from build123d import *

# Parameters (mm, degrees)
BASE_FLANGE1_DEPTH = 374.65
SKETCH6_R          = 3.3782
CUT_EXTRUDE1_DEPTH = 378.077201147
SKETCH7_R          = 4.3688
CUT_EXTRUDE2_DEPTH = 378.077201147
FILLET1_R          = 6.35


# Sheet-metal steps are written as plain solids
with BuildPart() as part:
    # Sketch1 → Base-Flange1 (new body)
    with BuildSketch(Plane(origin=(0, 0, 0), x_dir=(0, 0, -1), z_dir=(1, 0, 0))):
        with BuildLine():
            Line((0, 0), (25.4, 0))
            ThreePointArc((25.4, 0), (29.890128061, 1.859871939), (31.75, 6.35))
            Line((31.75, 6.35), (31.75, 31.75))
            Line((31.75, 31.75), (28.575, 31.75))
            Line((28.575, 31.75), (28.575, 6.35))
            ThreePointArc((28.575, 6.35), (27.64506403, 4.10493597), (25.4, 3.175))
            Line((25.4, 3.175), (0, 3.175))
            Line((0, 3.175), (0, 0))
        make_face()
    extrude(amount=BASE_FLANGE1_DEPTH)

    # Sketch6 → Cut-Extrude1 (cut, through all)
    with BuildSketch(Plane(origin=(0, 3.175, 0), x_dir=(1, 0, 0), z_dir=(0, 1, 0))):
        with Locations(Location((187.325, 11.1125, 0), (0, 0, 270))):
            Circle(SKETCH6_R)
        with Locations(Location((339.725, 11.1125, 0), (0, 0, 270))):
            Circle(SKETCH6_R)
        with Locations(Location((34.925, 11.1125, 0), (0, 0, 90))):
            Circle(SKETCH6_R)
    extrude(amount=-CUT_EXTRUDE1_DEPTH, mode=Mode.SUBTRACT)

    # Sketch7 → Cut-Extrude2 (cut, through all)
    with BuildSketch(Plane.XY.offset(-28.575)):
        with Locations((187.325, 20.6375)):
            Circle(SKETCH7_R)
        with Locations((339.725, 20.6375)):
            Circle(SKETCH7_R)
        with Locations(Location((34.925, 20.6375, 0), (0, 0, 180))):
            Circle(SKETCH7_R)
    extrude(amount=-CUT_EXTRUDE2_DEPTH, mode=Mode.SUBTRACT)

    # Fillet1
    fillet1_edges = [part.edges().sort_by_distance(p)[0] for p in [
        (374.65, 1.5875, 0),
        (0, 1.5875, 0),
        (374.65, 31.75, -30.1625),
        (0, 31.75, -30.1625),
    ]]
    fillet(fillet1_edges, radius=FILLET1_R)


solid = part.part
Verification items for the finished model (mm, model axes). A direction names the side the tool comes from. Round coordinates to 2 decimals unless told otherwise and drop trailing zeros. Write each loop counter-clockwise with the first axis right and the second up, starting at its lowest first coordinate (ties: lowest second). Pieces come first, ordered by that corner, then holes.
(1) Section check B-B (y = 11.5). Enter the section's corners in (x, z) (3 decimals), plus the area to 3 significant figures.
Returned:
outline: (0, -31.75) - (374.65, -31.75) - (374.65, -28.575) - (0, -28.575) - close
area: 1,190 mm2
(2) Material ranges on line 1 (Y direction, x = 308, z = -16.5) (3 decimals); line 2 (Z direction, x = 243, y = 8.5) (3 decimals); line 3 (Y direction, x = 27.5, z = -29), recorded low to high.
Returned:
line 1: y = 0 to 3.175
line 2: z = -31.75 to -28.575
line 3: y = 1.12 to 31.75
(3) Mould release check, pull along Z, two halves, no side actions. Record for faces 3 (the flat face through (185, 16, -28.575)), 4 (the flat face through (374.65, 3, -27)), 5 (the cylindrical face through (343.074, 1.61, -11.552)): pulls with the +Z half, pulls with the -Z half, needs draft (parallel to the pull), parting line crosses it, or undercut.
Returned:
face 3: pulls with the +Z half
face 4: needs draft
face 5: undercut
(4) Access from +Z, -Z, +X, -X, +Y, -Y to the whole of each face (thin tool, end or side, straight path). Record for faces 1 (the flat face through (0, 3, -27)), 2 (the flat face through (185, 3.175, -16)).
Returned:
face 1: +Z, -Z, -X, +Y, -Y
face 2: +Z, +X, -X, +Y
(5) Section check C-C (z = -19.5). Enter the section's corners in (x, y) (3 decimals).
Returned:
outline: (0, 0) - (374.65, 0) - (374.65, 3.175) - (0, 3.175) - close
(6) Depth check by flat-ended pin: pin 1 Ø12.5 at (x, z) = (262.5, -18) entering from +Y (3 decimals); pin 2 Ø14 at (x, y) = (187.32, 20.64) entering from +Z (3 decimals); pin 3 Ø1.5 at (x, z) = (230, -27) entering from -Y. Enter the tip coordinate at first touch or a pass-through.
Returned:
pin 1: stops at y = 3.175
pin 2: stops at z = -28.575
pin 3: stops at y = 0.06
(7) Section check A-A (x = 119). Enter the section's corners in (y, z) (3 decimals).
Returned:
outline: (0, -25.4) arc R6.35 ccw to (6.35, -31.75) - (31.75, -31.75) - (31.75, -28.575) - (6.35, -28.575) arc R3.175 cw to (3.175, -25.4) - (3.175, 0) - (0, 0) - close
